from build123d import *

# Parameters (mm, degrees)
CROQUIS1_W                                           = 150
CROQUIS1_H                                           = 150
SALIENTE_EXTRUIR1_DEPTH                              = 5
REDONDEO1_R                                          = 10
REDONDEO3_R                                          = 5
REFRENTADO_PARA_TORNILLO_CON_CABEZA_TRON_D           = 3.2639
REFRENTADO_PARA_TORNILLO_CON_CABEZA_TRON_DEPTH       = 50
REFRENTADO_PARA_TORNILLO_CON_CABEZA_TRON_CBORE_D     = 6.35
REFRENTADO_PARA_TORNILLO_CON_CABEZA_TRON_CBORE_DEPTH = 2.032
REFRENTADO_PARA_TORNILLO_CON_CABEZA_TRON_TIP         = 0.980574487


with BuildPart() as part:
    # Croquis1 → Saliente-Extruir1 (new body)
    with BuildSketch(Plane.XY):
        Rectangle(CROQUIS1_W, CROQUIS1_H)
    extrude(amount=SALIENTE_EXTRUIR1_DEPTH)

    # Redondeo1
    redondeo1_edges = [part.edges().sort_by_distance(p)[0] for p in [
        (75, -75, 2.5),
        (-75, -75, 2.5),
        (-75, 75, 2.5),
        (75, 75, 2.5),
    ]]
    fillet(redondeo1_edges, radius=REDONDEO1_R)

    # Redondeo3
    redondeo3_edges = [part.edges().sort_by_distance(p)[0] for p in [
        (72.071067812, 72.071067812, 5),
        (75, 0, 5),
        (72.071067812, -72.071067812, 5),
        (0, -75, 5),
        (-72.071067812, -72.071067812, 5),
        (-75, 0, 5),
        (-72.071067812, 72.071067812, 5),
        (0, 75, 5),
    ]]
    fillet(redondeo3_edges, radius=REDONDEO3_R - 0.0001)  # a hair under: the kernel refuses the full size

    # Refrentado para tornillo con cabeza troncocónica de #41
    with Locations(Plane.XY.offset(5)):
        with Locations((-70, 70), (-70, -70), (70, -70), (70, 70)):
            CounterBoreHole(REFRENTADO_PARA_TORNILLO_CON_CABEZA_TRON_D / 2, REFRENTADO_PARA_TORNILLO_CON_CABEZA_TRON_CBORE_D / 2, REFRENTADO_PARA_TORNILLO_CON_CABEZA_TRON_CBORE_DEPTH, depth=REFRENTADO_PARA_TORNILLO_CON_CABEZA_TRON_DEPTH)
            with Locations((0, 0, -(REFRENTADO_PARA_TORNILLO_CON_CABEZA_TRON_DEPTH + REFRENTADO_PARA_TORNILLO_CON_CABEZA_TRON_TIP / 2))):  # 118° drill point
                Cone(0, REFRENTADO_PARA_TORNILLO_CON_CABEZA_TRON_D / 2, REFRENTADO_PARA_TORNILLO_CON_CABEZA_TRON_TIP, mode=Mode.SUBTRACT)


solid = part.part
Design review of the part built by this model. Coordinates are the model's own, in mm. A direction names the side the tool comes from. Give positions to 0.01 mm unless a question says otherwise; leave off trailing zeros. Write each loop counter-clockwise with the first axis right and the second up, starting at its lowest first coordinate (ties: lowest second). Pieces come first, ordered by that corner, then holes. Notation, with made-up numbers: M 46.5,-11 L 73.5,-11 A25 cw 73.5,6 Z; hole C 66.5,37 d11. An arc over 180 degrees is marked long. Return JSON: item names as keys, results as strings. Group by question number.
Item 1: Clearance check with flat-ended pins moving along their axes: pin 1 Ø3 at (x, y) = (-70, -70) entering from -Z; pin 2 Ø3 at (x, y) = (70, -71.5) entering from +Z; pin 3 Ø2 at (x, z) = (-8.5, 2) entering from +Y; pin 4 Ø1.5 at (y, z) = (-3, 1.5) entering from +X. State where each tip first meets the part, or that it passes through.
Item 2: Tool access review of faces 1 (the cylindrical face through (-67.82, 67.69, 4)), 2 (the cylindrical face through (71.295, -70.993, 1.463)): name each direction out of +Z, -Z, +X, -X, +Y, -Y from which nothing blocks a thin tool from reaching the whole face with its end or side.
Item 3: The part is to be moulded in two halves that separate along X. For faces 3 (the flat face through (-1, 1, 0)), 4 (the cylindrical face through (-68.705, 69.007, 1.463)), 5 (the cylindrical face through (-73, -1, 4)), say which applies: pulls with the +X half, pulls with the -X half, needs draft (parallel to the pull), parting line crosses it, or undercut.
Item 4: Take a section at A-A (z = 2.2). Give the boundary of the cut face in (x, y).
Item 5: Wall thickness on line 1 along Y through (x, z) = (70, 1.95); line 2 along Y through (x, z) = (-70, 1.7): over which ranges is each line inside the solid? List them lowest first.
Return value:
{
 "1": {"pin 1": "passes through", "pin 2": "stops at z = 2.97", "pin 3": "stops at y = 74.9", "pin 4": "stops at x = 74.94"},
 "2": {"face 1": "+Z", "face 2": "+Z, -Z"},
 "3": {"face 3": "needs draft", "face 4": "undercut", "face 5": "pulls with the -X half"},
 "4": {"outline": "M -74.49,-65 A9.49 ccw -65,-74.49 L 65,-74.49 A9.49 ccw 74.49,-65 L 74.49,65 A9.49 ccw 65,74.49 L -65,74.49 A9.49 ccw -74.49,65 Z; hole C -70,-70 d3.26; hole C -70,70 d3.26; hole C 70,-70 d3.26; hole C 70,70 d3.26"},
 "5": {"line 1": "y = -73.2 to -71.63, -68.37 to 68.37, 71.63 to 73.2", "line 2": "y = -73.31 to -71.63, -68.37 to 68.37, 71.63 to 73.31"}
}
